Model file for the job. Use its own axes, mm. Round coordinates to 2 decimals unless told otherwise and drop trailing zeros. Loops run counter-clockwise (first coordinate to the right, second up) from the corner with the lowest first, then second, coordinate; pieces in that order, holes last. Notation, with made-up numbers: M 75,61 L 111,61 A19 cw 111,73 Z; hole C -36,16.5 d7. An arc over 180 degrees is marked long. Use a Markdown table: item, result. Add a question column.
Q1. Cut at A-A (z = 22.86). Give the cut face in (x, y), plus the area to 3 significant figures.
Q2. Probe line 1 (X direction, y = 1.8, z = 60.96); line 2 (X direction, y = 3.9, z = 22.5); line 3 (Z direction, x = 529.59, y = 2.85). List the from-to ranges inside material, lowest first. Write a range as from..to.
Q3. Mould opens along X. For faces 1 (the face through (525.365, 2.348, 20.662)), 2 (the face through (535.93, 2.35, 80.2)), 3 (the face through (266, 0, 41)), 4 (the face through (3.62, 2.35, 3.82)) say: +X half, -X half, draft (parallel to the pull), parting line (faces both ways), or undercut.
Q4. Pin check, flat tips, straight feed: pin 1 (2.5 mm diameter, centred on x = 3, y = 1.5, fed in from -Z); pin 2 (1.4 mm diameter, centred on x = 532.5, y = 2.5, fed in from -Z); pin 3 (1.4 mm diameter, centred on x = 537, y = 2.5, fed in from +Z); pin 4 (7.5 mm diameter, centred on x = 10.16, z = 22.86, fed in from -Y). Stop position of each tip, or through.
Q5. Cut at B-B (y = 0.75). State how many separate pieces and enclosed holes the cut face has, plus the area to 3 significant figures.
from build123d import *

# Parameters (mm, degrees)
SKETCH1_R           = 4.7625
BOSS_EXTRUDE1_DEPTH = 4.7625


with BuildPart() as part:
    # Sketch1 → Boss-Extrude1 (new body)
    with BuildSketch(Plane(origin=(0, 0, 0), x_dir=(1, 0, 0), z_dir=(0, 1, 0))):
        with BuildLine():
            Line((12.7, 0), (269.875, 0))
            Line((269.875, 0), (269.875, -83.82))
            Line((269.875, -83.82), (12.7, -83.82))
            ThreePointArc((12.7, -83.82), (3.719743879, -80.100256121), (0, -71.12))
            Line((0, -71.12), (0, -50.8))
            Line((0, -50.8), (10.16, -50.8))
            ThreePointArc((10.16, -50.8), (19.05, -41.91), (10.16, -33.02))
            Line((10.16, -33.02), (0, -33.02))
            Line((0, -33.02), (0, -12.7))
            ThreePointArc((0, -12.7), (3.719743879, -3.719743879), (12.7, 0))
        make_face()
        with Locations(Location((10.16, -60.96, 0), (0, 0, 90))):
            Circle(SKETCH1_R, mode=Mode.SUBTRACT)
        with Locations(Location((10.16, -22.86, 0), (0, 0, 90))):
            Circle(SKETCH1_R, mode=Mode.SUBTRACT)
    boss_extrude1 = extrude(amount=BOSS_EXTRUDE1_DEPTH)

    # Mirror1: Boss-Extrude1 across plane
    add(boss_extrude1.mirror(Plane(origin=(269.875, 4.7625, 0), x_dir=(0, 0, 1), z_dir=(-1, 0, 0))))


solid = part.part
Checked values:
| question | item | result |
|---|---|---|
| 1 | outline | M 0,0 L 5.4,0 L 5.4,4.76 L 0,4.76 Z; M 14.92,0 L 524.83,0 L 524.83,4.76 L 14.92,4.76 Z; M 534.35,0 L 539.75,0 L 539.75,4.76 L 534.35,4.76 Z |
| 1 | area | 2,480 mm^2 |
| 2 | line 1 | x = 0..5.4, 14.92..524.83, 534.35..539.75 |
| 2 | line 2 | x = 0..5.41, 14.91..524.84, 534.34..539.75 |
| 2 | line 3 | z = 0.26..18.1, 27.62..33.02, 50.8..56.2, 65.72..83.56 |
| 3 | face 1 | undercut |
| 3 | face 2 | +X half |
| 3 | face 3 | draft |
| 3 | face 4 | -X half |
| 4 | pin 1 | stops at z = 3.22 |
| 4 | pin 2 | stops at z = 0.92 |
| 4 | pin 3 | stops at z = 79.82 |
| 4 | pin 4 | passes through |
| 5 | separate pieces | 1 |
| 5 | enclosed holes | 4 |
| 5 | area | 44,200 mm^2 |
